from build123d import *

# Parameters (mm, degrees)
SKETCH1_W           = 14
SKETCH1_H           = 21
SKETCH1_R           = 1.55
SKETCH1_R_2         = 3.81
BOSS_EXTRUDE1_DEPTH = 2
FILLET1_R           = 2
SKETCH3_R           = 4.81
SKETCH3_R_2         = 3.81
BOSS_EXTRUDE2_DEPTH = 20
SKETCH4_R           = 4.81
SKETCH4_R_2         = 3.371204608
BOSS_EXTRUDE3_DEPTH = 2


with BuildPart() as part:
    # Sketch1 → Boss-Extrude1 (new body)
    with BuildSketch(Plane.XY):
        Rectangle(SKETCH1_W, SKETCH1_H)
        with Locations((0, 7.5)):
            Circle(SKETCH1_R, mode=Mode.SUBTRACT)
        with Locations(Location((0, -7.5, 0), (0, 0, 180))):
            Circle(SKETCH1_R, mode=Mode.SUBTRACT)
        Circle(SKETCH1_R_2, mode=Mode.SUBTRACT)
    extrude(amount=BOSS_EXTRUDE1_DEPTH)

    # Fillet1
    fillet1_edges = [part.edges().sort_by_distance(p)[0] for p in [
        (7, -10.5, 1),
        (-7, -10.5, 1),
        (-7, 10.5, 1),
        (7, 10.5, 1),
    ]]
    fillet(fillet1_edges, radius=FILLET1_R)

    # Sketch3 → Boss-Extrude2 (add)
    with BuildSketch(Plane.XY.offset(2)):
        with Locations(Location((0, 0, 0), (0, 0, 180))):
            Circle(SKETCH3_R)
        Circle(SKETCH3_R_2, mode=Mode.SUBTRACT)
    extrude(amount=BOSS_EXTRUDE2_DEPTH)

    # Sketch4 → Boss-Extrude3 (add)
    with BuildSketch(Plane.XY.offset(22)):
        with Locations(Location((0, 0, 0), (0, 0, 180))):
            Circle(SKETCH4_R)
        Circle(SKETCH4_R_2, mode=Mode.SUBTRACT)
    extrude(amount=BOSS_EXTRUDE3_DEPTH)


solid = part.part
Verification items for the finished model (mm, model axes). A direction names the side the tool comes from. Coordinates: 2 decimals unless noted, no trailing zeros. Order: outer loops, then holes, each group sorted by start corner. A loop starts at its lowest first (then second) coordinate and runs counter-clockwise, first axis right, second up. Notation, with made-up numbers: (67, -28) -> (75, -28) arc R32 cw to (75, 1) -> close; hole circle Ø5 at (-34.75, 33.5). An arc over 180 degrees is marked (long way). Put each result on its own line as item: value. Start each with the question number.
1. Mould release check, pull along X, two halves, no side actions. Record for faces 1 (the cylindrical face through (0.715, 6.125, 0.986)), 2 (the cylindrical face through (-2.22, 4.267, 12.846)), 3 (the flat face through (0, 10.5, 1)): released by +X, released by -X, zero draft, split by the parting line, or undercut.
2. Cross-section at C-C, the plane y = 0. Record the boundary of the cut face in (x, z), then the cut area to 3 significant figures.
3. Go/stop test with flat-tipped pins: pin 1 Ø3 at (x, y) = (0, 7.5) entering from +Z; pin 2 Ø1 at (y, z) = (3.5, 4) entering from +X; pin 3 Ø8 at (x, z) = (-1, 12) entering from +Y; pin 4 Ø4 at (x, y) = (-4.5, 5.5) entering from -Z. Record where each tip stops, or that it passes through.
4. Cross-section at A-A, the plane y = 7.5. Record the boundary of the cut face in (x, z), then the cut area to 3 significant figures.
5. Cross-section at B-B, the plane x = 2.75. Record the boundary of the cut face in (y, z), then the cut area to 3 significant figures.
6. Material ranges on L1, parallel to Y at x = 0, z = 0.6; L2, parallel to Y at x = 0, z = 8; L3, parallel to Z at x = 2.75, y = -9.5, recorded low to high. Write a range as [from, to].
7. Cross-section at D-D, the plane z = 20.25. Record the boundary of the cut face in (x, y).
8. Access from +Z, -Z, +X, -X, +Y, -Y to the whole of each face (thin tool, end or side, straight path). Record for faces 4 (the flat face through (0, 5, 2)), 5 (the cylindrical face through (-6.43, -9.9, 1.01)), 6 (the cylindrical face through (-0.83, -3.72, 10.85)).
Computed:
1. face 1: undercut
1. face 2: split by the parting line
1. face 3: zero draft
2. outline: (-7, 0) -> (-3.81, 0) -> (-3.81, 22) -> (-3.37, 22) -> (-3.37, 24) -> (-4.81, 24) -> (-4.81, 2) -> (-7, 2) -> close; (3.37, 22) -> (3.81, 22) -> (3.81, 0) -> (7, 0) -> (7, 2) -> (4.81, 2) -> (4.81, 24) -> (3.37, 24) -> close
2. area: 58.5 mm2
3. pin 1: through
3. pin 2: x = 3.76
3. pin 3: y = 4.81
3. pin 4: z = 0
4. outline: (-7, 0) -> (-1.55, 0) -> (-1.55, 2) -> (-7, 2) -> close; (1.55, 0) -> (7, 0) -> (7, 2) -> (1.55, 2) -> close
4. area: 21.8 mm2
5. outline: (-10.5, 0) -> (-2.64, 0) -> (-2.64, 22) -> (-1.95, 22) -> (-1.95, 24) -> (-3.95, 24) -> (-3.95, 2) -> (-10.5, 2) -> close; (1.95, 22) -> (2.64, 22) -> (2.64, 0) -> (10.5, 0) -> (10.5, 2) -> (3.95, 2) -> (3.95, 24) -> (1.95, 24) -> close
5. area: 91.8 mm2
6. L1: [-10.5, -9.05], [-5.95, -3.81], [3.81, 5.95], [9.05, 10.5]
6. L2: [-4.81, -3.81], [3.81, 4.81]
6. L3: [0, 2]
7. outline: circle Ø9.62 at (0, 0); hole circle Ø7.62 at (0, 0)
8. face 4: +Z
8. face 5: +Z, -Z, -X, -Y
8. face 6: -Z
